Geometry: final body of the model. Coordinates: model frame, mm. Coordinates: 2 decimals unless noted, no trailing zeros. Loops run counter-clockwise (first coordinate to the right, second up) from the corner with the lowest first, then second, coordinate; pieces in that order, holes last. Notation, with made-up numbers: M -33,19 L -24,19 A19 ccw -24,41 Z; hole C -1,20 d10. An arc over 180 degrees is marked long. Write each question's results on one line, items separated by ' | '. Start each with the question number.
from build123d import *

# Parameters (mm, degrees)
BOSS_EXTRUDE1_DEPTH = 3.4
SKETCH3_R           = 5
CUT_EXTRUDE1_DEPTH  = 6
CUT_EXTRUDE2_DEPTH  = 10
SKETCH6_R           = 35
CUT_EXTRUDE3_DEPTH  = 10
CUT_EXTRUDE4_DEPTH  = 1


with BuildPart() as part:
    # Sketch1 → Boss-Extrude1 (new body)
    with BuildSketch(Plane.XY):
        with BuildLine():
            Line((0, -30), (80, -30))
            Line((80, -30), (80, 5))
            Line((80, 5), (48, 5))
            Line((48, 5), (16.114075804, 25.304872277))
            ThreePointArc((16.114075804, 25.304872277), (-28.802310396, 8.392074585), (0, -30))
        make_face()
    extrude(amount=BOSS_EXTRUDE1_DEPTH)

    # Sketch3 → Cut-Extrude1 (cut)
    with BuildSketch(Plane.XY.offset(3.4)):
        Circle(SKETCH3_R)
    extrude(amount=-CUT_EXTRUDE1_DEPTH, mode=Mode.SUBTRACT)

    # Sketch5 → Cut-Extrude2 (cut)
    with BuildSketch(Plane.XY.offset(3.4)):
        with BuildLine():
            ThreePointArc((0, 10), (-8.660254038, 5), (-8.660254038, -5))
            ThreePointArc((-8.660254038, -5), (-10.124355653, -10.464101615), (-15.588457268, -9))
            ThreePointArc((-15.588457268, -9), (-15.588457268, 9), (0, 18))
            ThreePointArc((0, 18), (4, 14), (0, 10))
        make_face()
    extrude(amount=-CUT_EXTRUDE2_DEPTH, mode=Mode.SUBTRACT)

    # Sketch6 → Cut-Extrude3 (cut)
    with BuildSketch(Plane(origin=(0, 0, 0), x_dir=(-1, 0, 0), z_dir=(0, 0, -1))):
        Circle(SKETCH6_R)
    extrude(amount=-CUT_EXTRUDE3_DEPTH, mode=Mode.SUBTRACT)

    # Sketch7 → Cut-Extrude4 (cut)
    with BuildSketch(Plane.XY.offset(3.4)):
        Polygon((62.77538264, -14.5), (62.77538264, -21), (64.77538264, -21), (64.77538264, -14.5), (71.27538264, -14.5), (71.27538264, -12.5), (64.77538264, -12.5), (64.77538264, -6), (62.77538264, -6), (62.77538264, -12.5), (56.27538264, -12.5), (56.27538264, -14.5), align=None)
    extrude(amount=-CUT_EXTRUDE4_DEPTH, mode=Mode.SUBTRACT)


solid = part.part
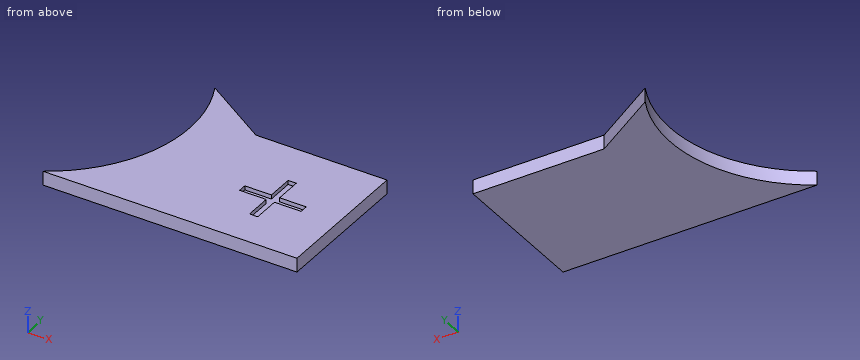
Item 1: Contact query for flat-ended pins moving along their axis: P1, Ø1.1, axis at x = 67, z = 3, coming from the +Y side; P2, Ø0.8, axis at y = -19, z = 3, coming from the -X side; P3, Ø2, axis at y = -21.5, z = 1, coming from the -X side. Output: stop coordinate, or through.
Item 2: Section D-D, the plane y = -13.5. Return loops of the section in (x, z).
Item 3: Ray query, L1, parallel to Y at x = 60, z = 2.8; L2, parallel to Y at x = 60.5, z = 0.5; L3, parallel to Y at x = 28, z = 2.2. Return the intervals inside material, ascending. Write a range as [from, to].
Item 4: Section A-A, the plane z = 0.95. Return loops of the section in (x, y).
Item 5: Section B-B, the plane y = -8.5. Return loops of the section in (x, z), plus the area to 3 significant figures.
Item 6: Section C-C, the plane x = 75. Return loops of the section in (y, z), plus the area to 3 significant figures.
Solutions:
1) P1: stops at y = 5 | P2: stops at x = 29.13 | P3: stops at x = 26.81
2) outline: M 32.29,0 L 80,0 L 80,3.4 L 71.28,3.4 L 71.28,2.4 L 56.28,2.4 L 56.28,3.4 L 32.29,3.4 Z
3) L1: y = [-30, -14.5], [-12.5, 5] | L2: y = [-30, 5] | L3: y = [-30, -21]
4) outline: M 18.03,-30 L 80,-30 L 80,5 L 48,5 L 31.32,15.62 A35 cw Z
5) outline: M 33.95,0 L 80,0 L 80,3.4 L 64.78,3.4 L 64.78,2.4 L 62.78,2.4 L 62.78,3.4 L 33.95,3.4 Z | area: 155 mm²
6) outline: M -30,0 L 5,0 L 5,3.4 L -30,3.4 Z | area: 119 mm²
